Could you check a few things on this model? Use its own coordinates, in mm. A direction names the side the tool comes from. Give positions to 0.01 mm unless a question says otherwise; leave off trailing zeros. Order: outer loops, then holes, each group sorted by start corner. A loop starts at its lowest first (then second) coordinate and runs counter-clockwise, first axis right, second up.
from build123d import *

# Parameters (mm, degrees)
SKETCH1_R            = 2.5
BOSS_EXTRUDE1_DEPTH  = 1
CUT_EXTRUDE2_DEPTH   = 0.1
CUT_EXTRUDE3_DEPTH   = 2
FILLET1_R            = 0.2
FILLET1_OF_MIRROR2_R = 0.2
CUT_EXTRUDE4_DEPTH   = 1
LPATTERN1_COUNT      = 2
LPATTERN1_PITCH      = 2.3
SKETCH5_W            = 3
SKETCH5_H            = 0.8
CUT_EXTRUDE5_DEPTH   = 0.5
CUT_EXTRUDE6_DEPTH   = 0.8
CUT_EXTRUDE7_REACH   = 51.52
CUT_EXTRUDE8_DEPTH   = 1
LPATTERN2_COUNT      = 2
LPATTERN2_PITCH      = 2.3
SKETCH9_W            = 3
SKETCH9_H            = 0.8
CUT_EXTRUDE9_DEPTH   = 0.5
CUT_EXTRUDE10_DEPTH  = 0.8
CUT_EXTRUDE11_REACH  = 51.52


with BuildPart() as part:
    # Sketch1 → Boss-Extrude1 (new, symmetric)
    with BuildSketch(Plane.XY):
        with BuildLine():
            Line((-7.5, 12.5), (7.5, 12.5))
            ThreePointArc((7.5, 12.5), (11.035533906, 11.035533906), (12.5, 7.5))
            Line((12.5, 7.5), (12.5, 7))
            ThreePointArc((12.5, 7), (12.939339828, 5.939339828), (14, 5.5))
            Line((14, 5.5), (46.5, 5.5))
            Line((46.5, 5.5), (46.5, -5.5))
            Line((46.5, -5.5), (14, -5.5))
            ThreePointArc((14, -5.5), (12.939339828, -5.939339828), (12.5, -7))
            Line((12.5, -7), (12.5, -7.5))
            ThreePointArc((12.5, -7.5), (11.035533906, -11.035533906), (7.5, -12.5))
            Line((7.5, -12.5), (-7.5, -12.5))
            ThreePointArc((-7.5, -12.5), (-11.035533906, -11.035533906), (-12.5, -7.5))
            Line((-12.5, -7.5), (-12.5, 7.5))
            ThreePointArc((-12.5, 7.5), (-11.035533906, 11.035533906), (-7.5, 12.5))
        make_face()
        with Locations((-6.5, -1.5)):
            Circle(SKETCH1_R, mode=Mode.SUBTRACT)
    extrude(amount=BOSS_EXTRUDE1_DEPTH, both=True)

    # Sketch2 → Cut-Extrude2 (cut)
    with BuildSketch(Plane.XY.offset(1)):
        with BuildLine():
            Line((11.5, 7), (11.5, 7.5))
            ThreePointArc((11.5, 7.5), (10.328427125, 10.328427125), (7.5, 11.5))
            Line((7.5, 11.5), (-7.5, 11.5))
            ThreePointArc((-7.5, 11.5), (-10.328427125, 10.328427125), (-11.5, 7.5))
            Line((-11.5, 7.5), (-11.5, -7.5))
            ThreePointArc((-11.5, -7.5), (-10.328427125, -10.328427125), (-7.5, -11.5))
            Line((-7.5, -11.5), (7.5, -11.5))
            ThreePointArc((7.5, -11.5), (10.328427125, -10.328427125), (11.5, -7.5))
            Line((11.5, -7.5), (11.5, -7))
            Line((11.5, -7), (11.5, 7))
        make_face()
    cut_extrude2 = extrude(amount=-CUT_EXTRUDE2_DEPTH, mode=Mode.SUBTRACT)

    # Mirror1: Cut-Extrude2 across plane
    add(cut_extrude2.mirror(Plane.XY), mode=Mode.SUBTRACT)

    # Sketch3 → Cut-Extrude3 (cut)
    with BuildSketch(Plane.XY.offset(1)):
        Polygon((19.5, 5.5), (19.5, 4), (21.5, 4), (22, 4.5), (46.5, 4.5), (46.5, 5.5), align=None)
    cut_extrude3 = extrude(amount=-CUT_EXTRUDE3_DEPTH, mode=Mode.SUBTRACT)

    # Fillet1
    fillet1_edges = [part.edges().sort_by_distance(p)[0] for p in [
        (19.5, 5.5, 0),
        (22, 4.5, 0),
    ]]
    fillet(fillet1_edges, radius=FILLET1_R)

    # Mirror2: Cut-Extrude3 across plane
    add(cut_extrude3.mirror(Plane.ZX), mode=Mode.SUBTRACT)

    # Fillet1 of Mirror2
    fillet1_of_mirror2_edges = [part.edges().sort_by_distance(p)[0] for p in [
        (19.5, -5.5, 0),
        (22, -4.5, 0),
    ]]
    fillet(fillet1_of_mirror2_edges, radius=FILLET1_OF_MIRROR2_R)

    # Sketch4 → Cut-Extrude4 (cut)
    with BuildSketch(Plane.XY.offset(1)):
        Polygon((46.5, -0.1), (19.5, -0.1), (14.5, -0.6), (14.5, -1.1), (19.5, -1.6), (46.5, -1.6), align=None)
    cut_extrude4 = extrude(amount=-CUT_EXTRUDE4_DEPTH, mode=Mode.SUBTRACT)

    # LPattern1: Cut-Extrude4 ×2
    with Locations(*[(0, -i * LPATTERN1_PITCH, 0) for i in range(1, LPATTERN1_COUNT)]):
        add(cut_extrude4, mode=Mode.SUBTRACT)

    # Sketch5 → Cut-Extrude5 (cut)
    with BuildSketch(Plane.XY.offset(1)):
        with Locations((24, -2)):
            Rectangle(SKETCH5_W, SKETCH5_H)
        with Locations((28.5, -2)):
            Rectangle(SKETCH5_W, SKETCH5_H)
    extrude(amount=-CUT_EXTRUDE5_DEPTH, mode=Mode.SUBTRACT)

    # Sketch6 → Cut-Extrude6 (cut)
    with BuildSketch(Plane.XZ.offset(2.4)):
        Polygon((35, 1), (31, 1), (32, 0), (34, 0), align=None)
        Polygon((43, 1), (39, 1), (40, 0), (42, 0), align=None)
    extrude(amount=-CUT_EXTRUDE6_DEPTH, mode=Mode.SUBTRACT)

    # Cut-Extrude7: up to this face of the body (flat: up to its plane)
    cut_extrude7_end = Plane(part.part.faces().sort_by_distance((33, -0.1, 0.5))[0])
    # Sketch7 → Cut-Extrude7 (cut, up to the picked face)
    with BuildSketch(Plane.XZ.offset(4.5), mode=Mode.PRIVATE) as cut_extrude7_sk1:
        Polygon((46.5, -1), (43.5, 1), (46.5, 1), align=None)
    cut_extrude7_tool1 = split(extrude(cut_extrude7_sk1.sketch, amount=-CUT_EXTRUDE7_REACH, mode=Mode.PRIVATE), bisect_by=cut_extrude7_end, keep=Keep.BOTH, mode=Mode.PRIVATE)
    add(cut_extrude7_tool1.solids().sort_by(Axis((45.5, -4.5, 0.333333), (0, 1, 0)))[0], mode=Mode.SUBTRACT)

    # Sketch8 → Cut-Extrude8 (cut)
    with BuildSketch(Plane(origin=(0, 0, -1), x_dir=(-1, 0, 0), z_dir=(0, 0, -1))):
        Polygon((-46.5, 0.1), (-19.5, 0.1), (-14.5, 0.6), (-14.5, 1.1), (-19.5, 1.6), (-46.5, 1.6), align=None)
    cut_extrude8 = extrude(amount=-CUT_EXTRUDE8_DEPTH, mode=Mode.SUBTRACT)

    # LPattern2: Cut-Extrude8 ×2
    with Locations(*[(0, i * LPATTERN2_PITCH, 0) for i in range(1, LPATTERN2_COUNT)]):
        add(cut_extrude8, mode=Mode.SUBTRACT)

    # Sketch9 → Cut-Extrude9 (cut)
    with BuildSketch(Plane(origin=(0, 0, -1), x_dir=(-1, 0, 0), z_dir=(0, 0, -1))):
        with Locations((-23, 2)):
            Rectangle(SKETCH9_W, SKETCH9_H)
        with Locations((-27.5, 2)):
            Rectangle(SKETCH9_W, SKETCH9_H)
    extrude(amount=-CUT_EXTRUDE9_DEPTH, mode=Mode.SUBTRACT)

    # Sketch10 → Cut-Extrude10 (cut)
    with BuildSketch(Plane(origin=(0, 2.4, 0), x_dir=(1, 0, 0), z_dir=(0, 1, 0))):
        Polygon((31, 1), (32, 0), (34, 0), (35, 1), align=None)
        Polygon((39, 1), (40, 0), (42, 0), (43, 1), align=None)
    extrude(amount=-CUT_EXTRUDE10_DEPTH, mode=Mode.SUBTRACT)

    # Cut-Extrude11: up to this face of the body (flat: up to its plane)
    cut_extrude11_end = Plane(part.part.faces().sort_by_distance((33, 0.1, -0.5))[0])
    # Sketch11 → Cut-Extrude11 (cut, up to the picked face)
    with BuildSketch(Plane(origin=(0, 4.5, 0), x_dir=(1, 0, 0), z_dir=(0, 1, 0)), mode=Mode.PRIVATE) as cut_extrude11_sk1:
        Polygon((46.5, -1), (43.5, 1), (46.5, 1), align=None)
    cut_extrude11_tool1 = split(extrude(cut_extrude11_sk1.sketch, amount=-CUT_EXTRUDE11_REACH, mode=Mode.PRIVATE), bisect_by=cut_extrude11_end, keep=Keep.BOTH, mode=Mode.PRIVATE)
    add(cut_extrude11_tool1.solids().sort_by(Axis((45.5, 4.5, -0.333333), (0, -1, 0)))[0], mode=Mode.SUBTRACT)


solid = part.part
Item 1: Imagine slicing it at A-A on x = -6.5. List the corners of the cut face in (y, z) for me.
Findings:
outline: (-12.5, -1) - (-11.5, -1) - (-11.5, -0.9) - (-4, -0.9) - (-4, 0.9) - (-11.5, 0.9) - (-11.5, 1) - (-12.5, 1) - close; (1, -0.9) - (11.5, -0.9) - (11.5, -1) - (12.5, -1) - (12.5, 1) - (11.5, 1) - (11.5, 0.9) - (1, 0.9) - close
Item 2: Imagine slicing it at C-C on y = 8.25. List the corners of the cut face in (x, z) for me.
Findings:
outline: (-12.44, -1) - (-11.43, -1) - (-11.43, -0.9) - (11.43, -0.9) - (11.43, -1) - (12.44, -1) - (12.44, 1) - (11.43, 1) - (11.43, 0.9) - (-11.43, 0.9) - (-11.43, 1) - (-12.44, 1) - close
Item 3: Please list where these lines run through material, in increasing order: line 1 along Y through (x, z) = (36.5, -0.35); line 2 along Y through (x, z) = (-6.5, -0.35); line 3 along Y through (x, z) = (17, 0.05).
Findings:
line 1: y = -4.5 to 0.1, 1.6 to 2.4, 3.9 to 4.5
line 2: y = -12.5 to -4, 1 to 12.5
line 3: y = -5.5 to -3.65, -2.65 to -1.35, -0.35 to 5.5
Item 4: Imagine slicing it at B-B on y = -9.75. List the corners of the cut face in (x, z) for me.
Findings:
outline: (-11.97, -1) - (-10.81, -1) - (-10.81, -0.9) - (10.81, -0.9) - (10.81, -1) - (11.97, -1) - (11.97, 1) - (10.81, 1) - (10.81, 0.9) - (-10.81, 0.9) - (-10.81, 1) - (-11.97, 1) - close
Item 5: We'd pull the mould along Y, two halves only. Please class faces 1 (the flat face through (43.5, 1.6, -0.4)), 2 (the flat face through (45, 2, 0)), 3 (the flat face through (42.5, 2, -0.5)): +Y half, -Y half, draft (parallel to the pull), parting line (faces both ways), or undercut.
Findings:
face 1: undercut
face 2: draft
face 3: undercut
Item 6: For pin 1 (10 mm diameter, centred on x = 2.5, y = -5, fed in from -Z); pin 2 (0.8 mm diameter, centred on x = 28, z = 0.5, fed in from +Y); pin 3 (0.6 mm diameter, centred on y = 2, z = -1, fed in from +X), each with a flat end and sliding along its axis, tell me the tip position at first contact or that it passes through.
Findings:
pin 1: stops at z = -0.9
pin 2: stops at y = 4.5
pin 3: stops at x = 43.95
Item 7: For faces 4 (the flat face through (0, 0, -0.9)), 5 (the flat face through (0, 0, 0.9)), 6 (the flat face through (43.5, -2.4, 0.4)), 7 (the flat face through (17.035, 2.646, -0.507)), which set-ups out of +Z, -Z, +X, -X, +Y, -Y let a thin tool reach every point of the face, with its end or its side?
Findings:
face 4: -Z
face 5: +Z
face 6: +Z, +X
face 7: -Z, +X
